from build123d import *

# Parameters (mm, degrees)
ENL_V_MAT_EXTRU_1_DEPTH = 1.3


with BuildPart() as part:
    # Esquisse1 → Révolution1 (revolve)
    with BuildSketch(Plane(origin=(0, 0, 0), x_dir=(0, 0, -1), z_dir=(1, 0, 0))):
        with BuildLine():
            Line((-2.4, 0), (-2.4, 1.4))
            ThreePointArc((-2.4, 1.4), (-2.024883171, 2.355248659), (-1.1, 2.8))
            Line((-1.1, 2.8), (0, 2.8))
            Line((0, 2.8), (0, 1.5))
            Line((0, 1.5), (16, 1.5))
            Line((16, 1.5), (16, 0))
            Line((16, 0), (-2.4, 0))
        make_face()
    revolve(axis=Axis((0, 0, 2.4), (0, 0, 1)))

    # Esquisse2 → Enlèv. mat.-Extru.1 (cut)
    with BuildSketch(Plane.XY.offset(2.4)):
        with BuildLine():
            ThreePointArc((-0.240728142, 1.210222096), (0, 1.4), (0.240728142, 1.210222096))
            ThreePointArc((0.240728142, 1.210222096), (0.499017901, 0.864324358), (0.927719008, 0.813587734))
            ThreePointArc((0.927719008, 0.813587734), (1.212435565, 0.7), (1.16844715, 0.396634361))
            ThreePointArc((1.16844715, 0.396634361), (0.998035801, 0), (1.16844715, -0.396634361))
            ThreePointArc((1.16844715, -0.396634361), (1.212435565, -0.7), (0.927719008, -0.813587734))
            ThreePointArc((0.927719008, -0.813587734), (0.499017901, -0.864324358), (0.240728142, -1.210222096))
            ThreePointArc((0.240728142, -1.210222096), (0, -1.4), (-0.240728142, -1.210222096))
            ThreePointArc((-0.240728142, -1.210222096), (-0.499017901, -0.864324358), (-0.927719008, -0.813587734))
            ThreePointArc((-0.927719008, -0.813587734), (-1.212435565, -0.7), (-1.16844715, -0.396634361))
            ThreePointArc((-1.16844715, -0.396634361), (-0.998035801, 0), (-1.16844715, 0.396634361))
            ThreePointArc((-1.16844715, 0.396634361), (-1.212435565, 0.7), (-0.927719008, 0.813587734))
            ThreePointArc((-0.927719008, 0.813587734), (-0.499017901, 0.864324358), (-0.240728142, 1.210222096))
        make_face()
    extrude(amount=-ENL_V_MAT_EXTRU_1_DEPTH, mode=Mode.SUBTRACT)


solid = part.part
Work out the finished part from the listing and answer in its coordinate system (mm). A direction names the side the tool comes from. Coordinates: 2 decimals unless noted, no trailing zeros. Write each loop counter-clockwise with the first axis right and the second up, starting at its lowest first coordinate (ties: lowest second). Pieces come first, ordered by that corner, then holes. Notation, with made-up numbers: M 75.25,-22.5 L 107.25,-22.5 A16 ccw 107.25,1.5 Z; hole C 35,-25 d1. An arc over 180 degrees is marked long. Use one line per item in the form item = value. Start each with the question number.
1. Each of these flat-tipped pins is pushed along its axis until it touches: P1, Ø3, axis at x = 0, z = -6, coming from the +Y side; P2, Ø1, axis at y = 1.5, z = -8.5, coming from the +X side. Where does it stop, or does it pass through?
2. The part is cut by section A-A (z = -2). Give the vertices of the cut face in (x, y), plus the area to 3 significant figures.
3. The mould has two halves that part along X. Classify faces 3 (the face through (1.2, 1.2, 0)), 4 (the face through (0, 0, 1.1)), 5 (the face through (-0.1, -2.8, 0.5)): released by +X, released by -X, zero draft, split by the parting line, or undercut.
4. A tool of negligible diameter and unlimited length cuts with its end or side. For faces 1 (the face through (0, 0, -16)), 2 (the face through (-0.07, -1.5, -8.11)), from which of +Z, -Z, +X, -X, +Y, -Y can it reach the whole face along a straight path? Write none if from no direction.
5. Straight lines are drawn through the part: probe 1 along Z at (x, y) = (-0.1, -1.25); probe 2 along Y at (x, z) = (0.1, -14.25); probe 3 along X at (y, z) = (-0.55, -13). For each, find the intervals that lie inside material, in ascending order. Write a range as from..to.
Evaluation:
q1.P1 = 1.5
q1.P2 = 1.12
q2.outline = C 0,0 d3
q2.area = 7.07 mm^2
q3.face_3 = zero draft
q3.face_4 = undercut
q3.face_5 = split by the parting line
q4.face_1 = -Z, +X, -X, +Y, -Y
q4.face_2 = -Z
q5.probe_1 = -16..1.1
q5.probe_2 = -1.5..1.5
q5.probe_3 = -1.4..1.4
